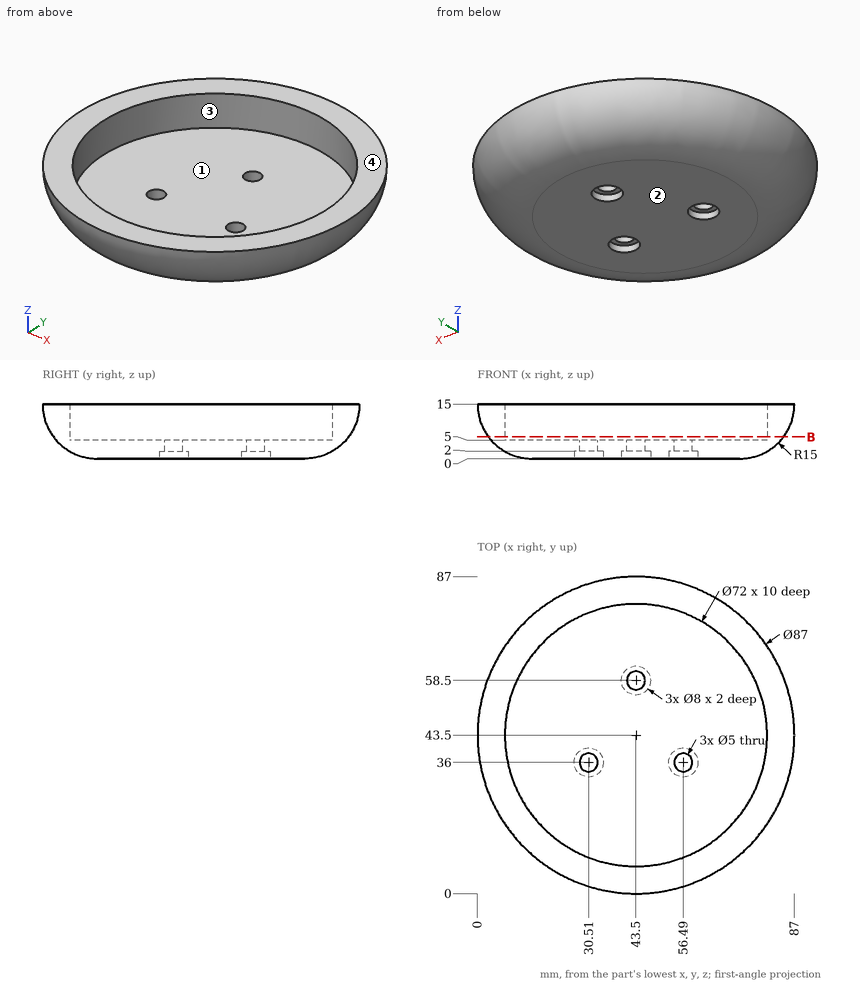
Source: three-view drawing plus pictorial views. Frame: mm from the lowest corner of the part. A direction names the side the tool comes from. Round coordinates to 2 decimals unless told otherwise and drop trailing zeros. Loops run counter-clockwise (first coordinate to the right, second up) from the corner with the lowest first, then second, coordinate; pieces in that order, holes last. Notation, with made-up numbers: M -39.5,67.25 L -35.5,67.25 A22 cw -35.5,89.25 Z; hole C 13.5,60.25 d11. An arc over 180 degrees is marked long. Answer as CSV lines item,"result". Start each with the question number.
(1) Draft query along Y for the marked faces 3 and 4. Return one class per face: released by +Y, released by -Y, zero draft, split by the parting line, or undercut.
(2) Section B-B, the plane z = 6. Output: boundary loops of the cut face in (x, y), plus the area to 3 significant figures.
(3) First-contact query: pin 1 (10.5 mm diameter, centred on x = 43.5, y = 58.5, fed in from +Z); pin 2 (4 mm diameter, centred on x = 48, z = 2.5, fed in from -Y) (1 decimal); pin 3 (1.5 mm diameter, centred on y = 30.5, z = 10.5, fed in from -X); pin 4 (4.5 mm diameter, centred on x = 56.49, y = 36, fed in from +Z). Flat tips, straight axial feed; report the tip coordinate or a pass-through.
(4) Line query: line 1 (X direction, y = 36, z = 1.3) (1 decimal); line 2 (Y direction, x = 52, z = 9.75) (1 decimal); line 3 (Y direction, x = 43.5, z = 1.2) (1 decimal). Output: solid intervals per line, ascending. Write a range as [from, to].
(5) Reachability of the marked faces 1 and 2 from +Z, -Z, +X, -X, +Y, -Y: full face, straight path, thin tool, end or side. Return the list, or none.
Values found:
1,face 3,"undercut"
1,face 4,"zero draft"
2,outline,"C 43.5,43.5 d81; hole C 43.5,43.5 d72"
2,area,"1,080 mm²"
3,pin 1,"stops at z = 5"
3,pin 2,"stops at y = 4.5"
3,pin 3,"stops at x = 2.38"
3,pin 4,"passes through"
4,line 1,"x = [9.7, 26.5], [34.5, 52.5], [60.5, 77.3]"
4,line 2,"y = [1.8, 8.5], [78.5, 85.2]"
4,line 3,"y = [9.1, 54.5], [62.5, 77.9]"
5,face 1,"+Z"
5,face 2,"-Z, +X, -X, +Y, -Y"
